Design review of the part built by this model. Coordinates are the model's own, in mm. A direction names the side the tool comes from. Give positions to 0.01 mm unless a question says otherwise; leave off trailing zeros. Loops run counter-clockwise (first coordinate to the right, second up) from the corner with the lowest first, then second, coordinate; pieces in that order, holes last. Notation, with made-up numbers: (18, 67.25) -> (23, 67.25) arc R26 ccw to (23, 102.25) -> close; hole circle Ø6 at (70, -8). An arc over 180 degrees is marked (long way). Use a Markdown table: item, result. Add a question column.
1. Add section C-C (z = -5). State the section outline as (x, y) points.
2. Add section A-A (x = -25). State the section outline as (y, z) points, and give its area (3 significant figures).
3. For faces 1 (the flat face through (-34, 2, 5)), 2 (the flat face through (-32, 7, 7.5)), 3 (the flat face through (-32, 7, 2.5)), 4 (the flat face through (-34, 12, 5)), list the 3-axis set-ups (+Z, -Z, +X, -X, +Y, -Y) from which the entire face can be reached by the end or side of a thin tool; tool diameter is ignored.
4. To check wall thickness, follow line 1 (Z direction, x = -5, y = 7.75); line 2 (Z direction, x = 28, y = 9.75); line 3 (X direction, y = 13.75, z = -31.5). State the ranges of each line that lie inside material, in increasing order.
5. Add section B-B (z = 5). State the section outline as (x, y) points.
6. For pin 1 Ø8 at (x, z) = (-35.5, 6.5) entering from -Y; pin 2 Ø1.5 at (y, z) = (10.5, -24) entering from +X; pin 3 Ø4 at (x, y) = (7.5, 11.5) entering from +Z, all flat-tipped, find the tip position at first contact; note any pin that passes through.
7. Draft analysis for pull direction X (two halves, no side actions). For faces 5 (the cylindrical face through (-36.9, 7.07, 9.88)), 6 (the cylindrical face through (-36.79, 7.07, 0.147)), 7 (the flat face through (-15, 7, 10)), 8 (the flat face through (39.8, 6.9, -27.6)), state which applies: pulls with the +X half, pulls with the -X half, needs draft (parallel to the pull), parting line crosses it, or undercut.
Autodesk Fusion 360 part; units mm, degrees
sketch "Sketch1" plane through (0, 0, 0) normal (0, 1, 0) x (1, 0, 0)
  line L0 (0, 0) -> (-30, 0)
  line L1 (-30, 0) -> (-30, -10)
  line L2 (-30, -10) -> (0, -10)
  line L3 (0, -10) -> (0, 0)
  line L4 (0, 0) -> (34.641, 20)
  line L5 (0, 0) -> (40, 0) construction
  line L6 (0, -10) -> (34.641, 10)
  line L7 (34.641, 10) -> (55, 35)
  line L8 (55, 35) -> (44.8205, 35)
  line L9 (44.8205, 35) -> (34.641, 20)
  dimension "d1" = 30
  dimension "d2" = 10
  dimension "d3" = 40
  dimension "d4" = 30
extrude "Extrude1" add sketch "Sketch1" along normal blind 14
sketch "Sketch2" plane through (-30, 0, 0) normal (-1, 0, 0) x (0, -1, 0)
  line L0 (0, 0) -> (0, 10)
  line L1 (0, 10) -> (-14, 10)
  line L2 (-14, 10) -> (-14, 0)
  line L3 (-14, 0) -> (0, 0)
sketch "Sketch3" plane through (-30, 0, 0) normal (-1, 0, 0) x (0, -1, 0)
  line L0 (-12, 7.5) -> (-2, 7.5)
  line L1 (-2, 7.5) -> (-2, 2.5)
  line L2 (-2, 2.5) -> (-12, 2.5)
  line L3 (-12, 2.5) -> (-12, 7.5)
  line L4 (-14, 10) -> (-14, 0)
  line L5 (0, 10) -> (-14, 10)
  dimension "d7" = 10
  dimension "d8" = 5
  dimension "d9" = 2
  dimension "d10" = 2.5
extrude "Extrude2" add sketch "Sketch3" along normal blind 5
cylinder "CylinderPrimitive1" add diameter 10 height -10 placed x (1, 0, 0) y (0, 0, -1) z (0, 1, 0) at (-37.9928, 12, 5)
sketch "Sketch5" plane through (0, 2, 0) normal (0, -1, 0) x (1, 0, 0)
  arc A0 (-33.6627, 7.5) -> (-33.6627, 2.5) centre (-37.9928, 5) ccw
  line L0 (-33.6627, 2.5) -> (-30, 2.5)
  line L1 (-30, 2.5) -> (-30, 7.5)
  line L2 (-30, 7.5) -> (-33.6627, 7.5)
  circle A1 centre (-37.9928, 5) radius 3.75
  dimension "d15" = 7.5
extrude "Extrude3" cut sketch "Sketch5" against normal blind 35 contours A1
ref_plane "WorkPlane1" through (-45, 7, 5) normal (-1, 0, 0) x (0, -1, 0)
sketch "Sketch6" plane through (-45, 7, 5) normal (-1, 0, 0) x (0, 1, 0)
  line L0 (13.2157, -10.5168) -> (-13.0296, -10.5168)
  line L1 (-13.0296, -10.5168) -> (-13.0296, 7.5386)
  line L2 (-13.0296, 7.5386) -> (13.2157, 7.5386)
  line L3 (13.2157, 7.5386) -> (13.2157, -10.5168)
extrude "Extrude4" cut sketch "Sketch6" against normal blind 4.25
sketch "Sketch7" plane through (0, 2, 0) normal (0, -1, 0) x (1, 0, 0)
  line L0 (-40.75, 2.4583) -> (-40.75, 0.8289)
  arc A0 (-40.75, 0.8289) -> (-33.6627, 2.5) centre (-37.9928, 5) ccw
  line L1 (-33.6627, 2.5) -> (-30, 2.5)
  line L2 (-30, 2.5) -> (-30, 7.5)
  line L3 (-30, 7.5) -> (-33.6627, 7.5)
  arc A1 (-33.6627, 7.5) -> (-40.75, 9.1711) centre (-37.9928, 5) ccw
  line L4 (-40.75, 9.1711) -> (-40.75, 7.5417)
  arc A2 (-40.75, 2.4583) -> (-40.75, 7.5417) centre (-37.9928, 5) ccw
Taken from the geometry:
| question | item | result |
|---|---|---|
| 1 | outline | (8.66, 0) -> (25.98, 0) -> (25.98, 14) -> (8.66, 14) -> close |
| 2 | outline | (0, 0) -> (14, 0) -> (14, 10) -> (0, 10) -> close |
| 2 | area | 140 mm^2 |
| 3 | face 1 | +Z, -Z, -X, -Y |
| 3 | face 2 | +Z, +Y, -Y |
| 3 | face 3 | -Z, +Y, -Y |
| 3 | face 4 | +Z, -Z, -X, +Y |
| 4 | line 1 | z = 0 to 10 |
| 4 | line 2 | z = -16.17 to -6.17 |
| 4 | line 3 | x = 42.45 to 52.15 |
| 5 | outline | (-34.24, 2) -> (-30, 2) -> (-30, 0) -> (8.66, 0) -> (8.66, 14) -> (-30, 14) -> (-30, 12) -> (-34.24, 12) -> close |
| 6 | pin 1 | stops at y = 2 |
| 6 | pin 2 | stops at x = 46.65 |
| 6 | pin 3 | stops at z = 6.82 |
| 7 | face 5 | undercut |
| 7 | face 6 | undercut |
| 7 | face 7 | needs draft |
| 7 | face 8 | pulls with the -X half |
